Design review of the part built by this model. Coordinates are the model's own, in mm. Round coordinates to 2 decimals unless told otherwise and drop trailing zeros. Order: outer loops, then holes, each group sorted by start corner. A loop starts at its lowest first (then second) coordinate and runs counter-clockwise, first axis right, second up.
from build123d import *

# Parameters (mm, degrees)
F0_W     = 139.7
F0_H     = 106.3625
F1_DEPTH = 19.05
F2_SIZE  = 5.08
F3_R     = 4.7625
F4_DEPTH = 10.16


with BuildPart() as f1:
    # F0 (on Top) → F1 (new body)
    with BuildSketch(Plane.XY):
        with Locations((69.85, -53.18125)):
            Rectangle(F0_W, F0_H)
    extrude(amount=F1_DEPTH)

    # F2
    f2_edges = [f1.edges().sort_by_distance(p)[0] for p in [
        (69.85, 0, 19.05),
        (0, -53.18125, 19.05),
        (69.85, -106.3625, 19.05),
        (139.7, -53.18125, 19.05),
    ]]
    chamfer(f2_edges, length=F2_SIZE)

    # F3 (on face) → F4 (cut)
    with BuildSketch(Plane.XY.offset(19.05)):
        with Locations((41.5925, -45.72)):
            Circle(F3_R)
        with Locations((105.0925, -45.72)):
            Circle(F3_R)
    extrude(amount=-F4_DEPTH, mode=Mode.SUBTRACT)


solid = f1.part
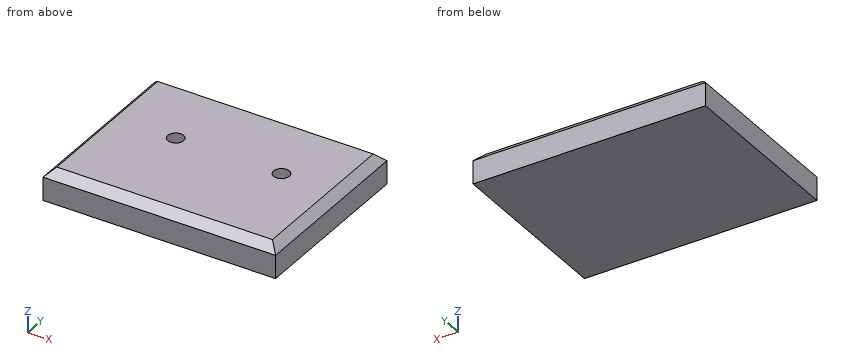
1) To check wall thickness, follow line 1 along X through (y, z) = (-60, 14); line 2 along X through (y, z) = (-49, 13.5); line 3 along Z through (x, y) = (87, -102). State the ranges of each line that lie inside material, in increasing order.
Results:
line 1: x = 0.03 to 139.67
line 2: x = 0 to 38.14, 45.05 to 101.64, 108.55 to 139.7
line 3: z = 0 to 18.33
2) Take a section at B-B on y = -45.72. Give the boundary of the cut face in (x, z) (3 decimals), plus the area to 3 significant figures.
Results:
outline: (0, 0) - (139.7, 0) - (139.7, 13.97) - (134.62, 19.05) - (109.855, 19.05) - (109.855, 8.89) - (100.33, 8.89) - (100.33, 19.05) - (46.355, 19.05) - (46.355, 8.89) - (36.83, 8.89) - (36.83, 19.05) - (5.08, 19.05) - (0, 13.97) - close
area: 2,440 mm2
3) Clearance check with a flat-ended pin moving along its axis: P1, Ø3, axis at x = 103, y = -47, coming from the +Z side. State where the tip first meets the part, or that it passes through.
Results:
P1: stops at z = 8.89
4) Take a section at A-A on z = 17. Give the boundary of the cut face in (x, y) (1 decimal), plus the area to 3 significant figures.
Results:
outline: (3, -103.3) - (136.7, -103.3) - (136.7, -3) - (3, -3) - close; hole circle Ø9.5 at (41.6, -45.7); hole circle Ø9.5 at (105.1, -45.7)
area: 13,300 mm2
